Read the model definition and answer for the solid it produces. Units are mm, in the model's axes. A direction names the side the tool comes from. Round coordinates to 2 decimals unless told otherwise and drop trailing zeros. Order: outer loops, then holes, each group sorted by start corner. A loop starts at its lowest first (then second) coordinate and runs counter-clockwise, first axis right, second up.
from build123d import *

# Parameters (mm, degrees)
SKETCH1_R                                       = 1.725
BOSS_EXTRUDE1_DEPTH                             = 2
SKETCH2_R                                       = 1
SKETCH2_R_2                                     = 1.725
BOSS_EXTRUDE2_DEPTH                             = 3
SKETCH3_R                                       = 6.225
CUT_EXTRUDE1_DEPTH                              = 2.4
CSK_FOR_M3_FLAT_HEAD_MACHINE_SCREW2_D           = 3.6
CSK_FOR_M3_FLAT_HEAD_MACHINE_SCREW2_CSINK_D     = 6.3
CSK_FOR_M3_FLAT_HEAD_MACHINE_SCREW2_CSINK_ANGLE = 90
CSK_FOR_M2_FLAT_HEAD_MACHINE_SCREW1_D           = 2.6
CSK_FOR_M2_FLAT_HEAD_MACHINE_SCREW1_CSINK_D     = 4.4
CSK_FOR_M2_FLAT_HEAD_MACHINE_SCREW1_CSINK_ANGLE = 90
FILLET1_R                                       = 2


with BuildPart() as part:
    # Sketch1 → Boss-Extrude1 (new body)
    with BuildSketch(Plane.XY):
        with BuildLine():
            Line((10, 4), (-8, 4))
            Line((-8, 4), (-8, 3.010972637))
            Line((-8, 3.010972637), (0.218908182, 2.189081818))
            ThreePointArc((0.218908182, 2.189081818), (2.2, 0), (0.218908182, -2.189081818))
            Line((0.218908182, -2.189081818), (-8, -3.010972637))
            Line((-8, -3.010972637), (-8, -4))
            Line((-8, -4), (10, -4))
            ThreePointArc((10, -4), (14, 0), (10, 4))
        make_face()
        with Locations((10, 0)):
            Circle(SKETCH1_R, mode=Mode.SUBTRACT)
    extrude(amount=BOSS_EXTRUDE1_DEPTH)

    # Sketch2 → Boss-Extrude2 (add)
    with BuildSketch(Plane.XY.offset(2)):
        with BuildLine():
            Line((-8, 4), (-8, -4))
            Line((-8, -4), (10, -4))
            ThreePointArc((10, -4), (14, 0), (10, 4))
            Line((10, 4), (-8, 4))
        make_face()
        Circle(SKETCH2_R, mode=Mode.SUBTRACT)
        with Locations((10, 0)):
            Circle(SKETCH2_R_2, mode=Mode.SUBTRACT)
    extrude(amount=BOSS_EXTRUDE2_DEPTH)

    # Sketch3 → Cut-Extrude1 (cut)
    with BuildSketch(Plane(origin=(0, 0, 0), x_dir=(-1, 0, 0), z_dir=(0, 0, -1))):
        with Locations((-10, 0)):
            Circle(SKETCH3_R)
    extrude(amount=-CUT_EXTRUDE1_DEPTH, mode=Mode.SUBTRACT)

    # CSK for M3 Flat Head Machine Screw2 (through all)
    with Locations(Plane(origin=(10, 0, 5), x_dir=(1, 0, 0), z_dir=(0, 0, 1))):
        with Locations((0, 0)):
            CounterSinkHole(CSK_FOR_M3_FLAT_HEAD_MACHINE_SCREW2_D / 2, CSK_FOR_M3_FLAT_HEAD_MACHINE_SCREW2_CSINK_D / 2, counter_sink_angle=CSK_FOR_M3_FLAT_HEAD_MACHINE_SCREW2_CSINK_ANGLE)

    # CSK for M2 Flat Head Machine Screw1 (through all)
    with Locations(Plane.XY.offset(5)):
        with Locations((0, 0)):
            CounterSinkHole(CSK_FOR_M2_FLAT_HEAD_MACHINE_SCREW1_D / 2, CSK_FOR_M2_FLAT_HEAD_MACHINE_SCREW1_CSINK_D / 2, counter_sink_angle=CSK_FOR_M2_FLAT_HEAD_MACHINE_SCREW1_CSINK_ANGLE)

    # Fillet1
    fillet1_edges = [part.edges().sort_by_distance(p)[0] for p in [
        (5.230238476, 4, 1.2),
        (5.230238476, -4, 1.2),
        (-8, -4, 2.5),
        (-8, 4, 2.5),
    ]]
    fillet(fillet1_edges, radius=FILLET1_R)


solid = part.part
Q1. A cutting plane is placed at A-A, the plane y = 0. Give the vertices of the cut face in (x, z) (3 decimals), plus the area to 3 significant figures.
Outcome:
outline: (-8, 2) - (-1.3, 2) - (-1.3, 4.1) - (-2.2, 5) - (-8, 5) - close; (1.3, 2) - (2.2, 2) - (2.2, 0) - (3.775, 0) - (3.775, 2.4) - (8.2, 2.4) - (8.2, 3.65) - (6.85, 5) - (2.2, 5) - (1.3, 4.1) - close; (11.8, 2.4) - (14, 2.4) - (14, 5) - (13.15, 5) - (11.8, 3.65) - close
area: 45.3 mm2
Q2. A cutting plane is placed at C-C, the plane x = 0. Give the vertices of the cut face in (y, z), plus the area to 3 significant figures.
Outcome:
outline: (-4, 0) - (-2.21, 0) - (-2.21, 2) - (-1.3, 2) - (-1.3, 4.1) - (-2.2, 5) - (-4, 5) - close; (1.3, 2) - (2.21, 2) - (2.21, 0) - (4, 0) - (4, 5) - (2.2, 5) - (1.3, 4.1) - close
area: 22.5 mm2
Q3. A cutting plane is placed at D-D, the plane z = 1.15. Give the vertices of the cut face in (x, y) (3 decimals), plus the area to 3 significant figures.
Outcome:
outline: (-7.741, -2.985) arc R2 ccw to (-6, -4) - (2.022, -4) arc R2 ccw to (3.962, -1.514) arc R6.225 cw to (3.962, 1.514) arc R2 ccw to (2.022, 4) - (-6, 4) arc R2 ccw to (-7.741, 2.985) - (0.219, 2.189) arc R2.2 cw to (0.219, -2.189) - close
area: 43.0 mm2
Q4. Flat-ended cylindrical pins translate along their axes: pin 1 (3 mm diameter, centred on x = 10, y = 0, fed in from -Z); pin 2 (2.5 mm diameter, centred on x = 9, y = -1.5, fed in from -Z); pin 3 (3 mm diameter, centred on x = -2.5, y = -0.5, fed in from -Z). Find the tip coordinate at first contact, or state that the pin passes through.
Outcome:
pin 1: passes through
pin 2: stops at z = 2.4
pin 3: stops at z = 2
Q5. For a pull along Y with two mould halves and no side action, classify faces 1 (the face through (3, 0, 5)), 2 (the face through (0.17, 1.29, 3.04)), 3 (the face through (-7.2, 3.6, 2.5)), 4 (the face through (-4, 0, 2)) as released by +Y, released by -Y, zero draft, split by the parting line, or undercut.
Outcome:
face 1: zero draft
face 2: undercut
face 3: released by +Y
face 4: undercut
Q6. For faces 5 (the face through (-8, 0, 3)), 6 (the face through (2.2, 0, 1)), determine the directions among +Z, -Z, +X, -X, +Y, -Y from which every point of the face is accessible in a straight line to the end or side of a thin tool.
Outcome:
face 5: +Z, -Z, -X, +Y, -Y
face 6: -Z, -X
Q7. A cutting plane is placed at B-B, the plane z = 3.25. Give the vertices of the cut face in (x, y), plus the area to 3 significant figures.
Outcome:
outline: (-8, -2) arc R2 ccw to (-6, -4) - (10, -4) arc R4 ccw to (10, 4) - (-6, 4) arc R2 ccw to (-8, 2) - close; hole circle Ø2.6 at (0, 0); hole circle Ø3.6 at (10, 0)
area: 152 mm2
Q8. Straight lines are drawn through the part: probe 1 along X at (y, z) = (0, 3.55); probe 2 along Y at (x, z) = (0, 2.85); probe 3 along Y at (x, z) = (10, 2.85). For each, find the intervals that lie inside material, in ascending order.
Outcome:
probe 1: x = -8 to -1.3, 1.3 to 8.2, 11.8 to 14
probe 2: y = -4 to -1.3, 1.3 to 4
probe 3: y = -4 to -1.8, 1.8 to 4
